The listing builds one solid part. Answer for the finished solid, in the listing's coordinates (mm). Give positions to 0.01 mm unless a question says otherwise; leave off trailing zeros. Loops run counter-clockwise (first coordinate to the right, second up) from the corner with the lowest first, then second, coordinate; pieces in that order, holes last. Notation, with made-up numbers: M 19.25,-8.75 L 62.25,-8.75 A29 ccw 62.25,25.25 Z; hole C -1,63.25 d9. An arc over 180 degrees is marked long. Return JSON: item names as keys, results as strings.
from build123d import *

# Parameters (mm, degrees)
SKETCH_1_W                  = 20
SKETCH_1_H                  = 20
SKETCH_1_W_2                = 18
SKETCH_1_H_2                = 18
EXTRUDE_1_DEPTH             = 160
HOLE_WIZARD_5_0_5_1_REACH   = 163.555
HOLE_WIZARD_5_0_5_1_BORE_R  = 2.5
PATTERN_LINEAR_1_COUNT      = 2
PATTERN_LINEAR_1_PITCH      = 50
MIRROR_1_COPY_1_REACH       = 163.555
MIRROR_1_COPY_1_SKETCH_R    = 2.5
HOLE_WIZARD_4_0_4_1_D       = 4
HOLE_WIZARD_13_0_13_1_D     = 13
HOLE_WIZARD_13_0_13_1_DEPTH = 1


with BuildPart() as part:
    # Sketch 1 → Extrude 1 (new, symmetric)
    with BuildSketch(Plane.XY):
        Rectangle(SKETCH_1_W, SKETCH_1_H)
        Rectangle(SKETCH_1_W_2, SKETCH_1_H_2, mode=Mode.SUBTRACT)
    extrude(amount=EXTRUDE_1_DEPTH, both=True)

    # Hole Wizard 5.0 _5_ _1 bore → Hole Wizard 5.0 _5_ _1 (cut, up to next)
    with BuildSketch(Plane(origin=(0, -10, 0), x_dir=(-1, 0, 0), z_dir=(0, -1, 0)), mode=Mode.PRIVATE) as hole_wizard_5_0_5_1_sk1:
        with Locations((-2.5, 145.9)):
            Circle(HOLE_WIZARD_5_0_5_1_BORE_R)
    hole_wizard_5_0_5_1_tool1 = extrude(hole_wizard_5_0_5_1_sk1.sketch, amount=-HOLE_WIZARD_5_0_5_1_REACH, mode=Mode.PRIVATE) & part.part
    # Hole Wizard 5.0 _5_ _1 bore → Hole Wizard 5.0 _5_ _1 (cut, up to next)
    with BuildSketch(Plane(origin=(0, -10, 0), x_dir=(-1, 0, 0), z_dir=(0, -1, 0)), mode=Mode.PRIVATE) as hole_wizard_5_0_5_1_sk2:
        with Locations((-2.5, 120.9)):
            Circle(HOLE_WIZARD_5_0_5_1_BORE_R)
    hole_wizard_5_0_5_1_tool2 = extrude(hole_wizard_5_0_5_1_sk2.sketch, amount=-HOLE_WIZARD_5_0_5_1_REACH, mode=Mode.PRIVATE) & part.part
    hole_wizard_5_0_5_1_1 = hole_wizard_5_0_5_1_tool1.solids().sort_by_distance((2.5, -10, -145.9))[0]
    add(hole_wizard_5_0_5_1_1, mode=Mode.SUBTRACT)
    hole_wizard_5_0_5_1_2 = hole_wizard_5_0_5_1_tool2.solids().sort_by_distance((2.5, -10, -120.9))[0]
    add(hole_wizard_5_0_5_1_2, mode=Mode.SUBTRACT)
    hole_wizard_5_0_5_1 = hole_wizard_5_0_5_1_1 + hole_wizard_5_0_5_1_2  # Hole Wizard 5.0 _5_ _1 as one shape, for the pattern or mirror that repeats it

    # Pattern Linear 1: Hole Wizard 5.0 _5_ _1 ×2
    with Locations(*[(0, 0, i * PATTERN_LINEAR_1_PITCH) for i in range(1, PATTERN_LINEAR_1_COUNT)]):
        add(hole_wizard_5_0_5_1, mode=Mode.SUBTRACT)

    # Mirror 1: Hole Wizard 5.0 _5_ _1 across plane
    add(hole_wizard_5_0_5_1.mirror(Plane(origin=(0, 0, 0), x_dir=(1, 0, 0), z_dir=(0, 0, -1))), mode=Mode.SUBTRACT)

    # Mirror 1 copy 1 sketch → Mirror 1 copy 1 (cut, up to next)
    with BuildSketch(Plane(origin=(0, -10, -50), x_dir=(-1, 0, 0), z_dir=(0, -1, 0)), mode=Mode.PRIVATE) as mirror_1_copy_1_sk1:
        with Locations((-2.5, -145.9)):
            Circle(MIRROR_1_COPY_1_SKETCH_R)
    mirror_1_copy_1_tool1 = extrude(mirror_1_copy_1_sk1.sketch, amount=-MIRROR_1_COPY_1_REACH, mode=Mode.PRIVATE) & part.part
    # Mirror 1 copy 1 sketch → Mirror 1 copy 1 (cut, up to next)
    with BuildSketch(Plane(origin=(0, -10, -50), x_dir=(-1, 0, 0), z_dir=(0, -1, 0)), mode=Mode.PRIVATE) as mirror_1_copy_1_sk2:
        with Locations((-2.5, -120.9)):
            Circle(MIRROR_1_COPY_1_SKETCH_R)
    mirror_1_copy_1_tool2 = extrude(mirror_1_copy_1_sk2.sketch, amount=-MIRROR_1_COPY_1_REACH, mode=Mode.PRIVATE) & part.part
    add(mirror_1_copy_1_tool1.solids().sort_by_distance((2.5, -10, 95.9))[0], mode=Mode.SUBTRACT)
    add(mirror_1_copy_1_tool2.solids().sort_by_distance((2.5, -10, 70.9))[0], mode=Mode.SUBTRACT)

    # Hole Wizard 4.0 _4_ _1 (through all)
    with Locations(Plane(origin=(0, -10, 0), x_dir=(-1, 0, 0), z_dir=(0, -1, 0))):
        with Locations((0, -108)):
            hole_wizard_4_0_4_1 = Hole(HOLE_WIZARD_4_0_4_1_D / 2)

    # Mirror 2: Hole Wizard 4.0 _4_ _1 across plane
    add(hole_wizard_4_0_4_1.mirror(Plane(origin=(0, 0, 0), x_dir=(1, 0, 0), z_dir=(0, 0, -1))), mode=Mode.SUBTRACT)

    # Hole Wizard 13.0 _13_ _1
    with Locations(Plane(origin=(0, 9, 0), x_dir=(-1, 0, 0), z_dir=(0, -1, 0))):
        with Locations((-2.5, 145.9), (-2.5, 120.9), (-2.5, 95.9), (-2.5, 70.9)):
            hole_wizard_13_0_13_1 = Hole(HOLE_WIZARD_13_0_13_1_D / 2, depth=HOLE_WIZARD_13_0_13_1_DEPTH)

    # Mirror 3: Hole Wizard 13.0 _13_ _1 across plane
    add(hole_wizard_13_0_13_1.mirror(Plane(origin=(0, 0, 0), x_dir=(1, 0, 0), z_dir=(0, 0, -1))), mode=Mode.SUBTRACT)


solid = part.part
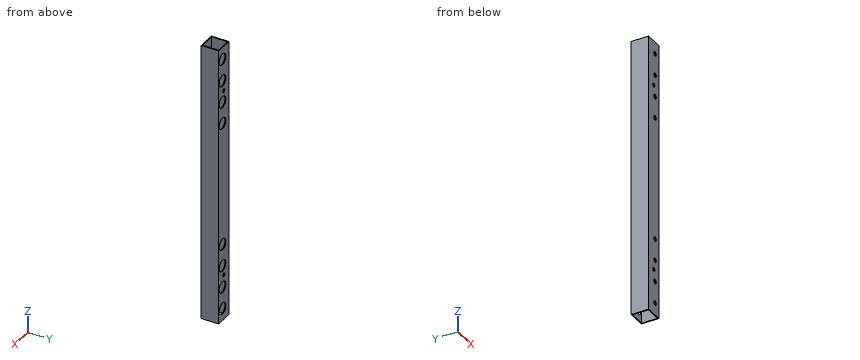
(1) Straight lines are drawn through the part: line 1 along X through (y, z) = (-9.7, 145.9); line 2 along X through (y, z) = (-3.75, -61). For each, find the intervals that lie inside material, in ascending order.
Values follow:
{"line 1": "-10 to 0, 5 to 10", "line 2": "-10 to -9, 9 to 10"}
(2) The part is cut by section A-A (y = 3.75). Determine the outline of the cut face in (x, z).
Values follow:
{"outline": "M -10,-160 L -9,-160 L -9,160 L -10,160 Z; M 9,-160 L 10,-160 L 10,160 L 9,160 Z"}
(3) The part is cut by section B-B (z = 36.5). Determine the outline of the cut face in (x, y), and give its area (3 significant figures).
Values follow:
{"outline": "M -10,-10 L 10,-10 L 10,10 L -10,10 Z; hole M -9,-9 L 9,-9 L 9,9 L -9,9 Z", "area": "76.0 mm²"}
(4) Given pin 1 (11.5 mm diameter, centred on x = 2.5, z = 120.9, fed in from -Y); pin 2 (10.5 mm diameter, centred on x = 2.5, z = -145.9, fed in from +Y), each flat-ended and moving along its own axis, determine where each tip first touches the part or whether it passes through.
Values follow:
{"pin 1": "y = -10", "pin 2": "y = -9"}
